```python
from build123d import *

# Parameters (mm, degrees)
SZKIC1_W                    = 30.3
SZKIC1_H                    = 11.1
SZKIC1_W_2                  = 28.304453741
SZKIC1_H_2                  = 9.1
DODANIE_WYCI_GNI_CIE1_DEPTH = 2
SZKIC2_W                    = 32.5
SZKIC2_H                    = 13.3
DODANIE_WYCI_GNI_CIE2_DEPTH = 1
ZAOKR_GLENIE1_R             = 0.5
SZKIC3_W                    = 1.095546259
SZKIC3_H                    = 0.5
SZKIC3_W_2                  = 1.2
SZKIC3_W_3                  = 0.5
SZKIC3_H_2                  = 1.2
SZKIC3_H_3                  = 1.1
WYTNIJ_WYCI_GNI_CIE1_DEPTH  = 1.4
ZAOKR_GLENIE2_R             = 0.5
SZKIC4_W                    = 2
SZKIC4_H                    = 1.15
SZKIC4_W_2                  = 1.145546259
SZKIC4_H_2                  = 2
SZKIC4_W_3                  = 1.15
DODANIE_WYCI_GNI_CIE3_DEPTH = 0.9
SZKIC5_W                    = 0.9
SZKIC5_H                    = 2
DODANIE_WYCI_GNI_CIE4_DEPTH = 0.5
SZKIC6_W                    = 2
SZKIC6_H                    = 0.9
DODANIE_WYCI_GNI_CIE5_DEPTH = 0.5
SZKIC7_W                    = 0.9
SZKIC7_H                    = 2
DODANIE_WYCI_GNI_CIE6_DEPTH = 0.5
ZAOKR_GLENIE5_R             = 1
SZKIC8_W                    = 28.304453741
SZKIC8_H                    = 9.1
DODANIE_WYCI_GNI_CIE7_DEPTH = 0.6
SZKIC9_W                    = 15.3
SZKIC9_H                    = 5.1
WYTNIJ_WYCI_GNI_CIE2_DEPTH  = 1.6
SZKIC10_W                   = 15.3
SZKIC10_H                   = 5.1
DODANIE_WYCI_GNI_CIE8_DEPTH = 2.5
ZAOKR_GLENIE6_R             = 0.4
SZKIC11_W                   = 2
SZKIC11_H                   = 5.1
WYTNIJ_WYCI_GNI_CIE3_DEPTH  = 0.3


with BuildPart() as part:
    # Szkic1 → Dodanie-wyciągnięcie1 (new body)
    with BuildSketch(Plane.XY):
        with Locations((-1.679789747, 1.465189223)):
            Rectangle(SZKIC1_W, SZKIC1_H)
        with Locations((-1.682016617, 1.465189223)):
            Rectangle(SZKIC1_W_2, SZKIC1_H_2, mode=Mode.SUBTRACT)
    extrude(amount=DODANIE_WYCI_GNI_CIE1_DEPTH)

    # Szkic2 → Dodanie-wyciągnięcie2 (add)
    with BuildSketch(Plane.XY.offset(2)):
        with Locations((-1.679789747, 1.465189223)):
            Rectangle(SZKIC2_W, SZKIC2_H)
    extrude(amount=DODANIE_WYCI_GNI_CIE2_DEPTH)

    # Zaokrąglenie1
    zaokr_glenie1_edges = [part.edges().sort_by_distance(p)[0] for p in [
        (-17.929789747, 1.465189223, 3),
        (-1.679789747, -5.184810777, 3),
        (14.570210253, 1.465189223, 3),
        (-1.679789747, 8.115189223, 3),
    ]]
    fillet(zaokr_glenie1_edges, radius=ZAOKR_GLENIE1_R)

    # Szkic3 → Wytnij-wyciągnięcie1 (cut)
    with BuildSketch(Plane(origin=(0, 0, 0), x_dir=(-1, 0, 0), z_dir=(0, 0, -1))):
        with Locations((16.382016617, 2.715189223)):
            Rectangle(SZKIC3_W, SZKIC3_H)
        with Locations((-13.070210253, 0.215189223)):
            Rectangle(SZKIC3_W_2, SZKIC3_H)
        with Locations((2.932016617, 6.615189223)):
            Rectangle(SZKIC3_W_3, SZKIC3_H_2)
        with Locations((0.432016617, 6.615189223)):
            Rectangle(SZKIC3_W_3, SZKIC3_H_2)
        with Locations((-13.070210253, 2.715189223)):
            Rectangle(SZKIC3_W_2, SZKIC3_H)
        with Locations((2.932016617, -3.634810777)):
            Rectangle(SZKIC3_W_3, SZKIC3_H_3)
        with Locations((0.432016617, -3.634810777)):
            Rectangle(SZKIC3_W_3, SZKIC3_H_3)
        with Locations((16.382016617, 0.215189223)):
            Rectangle(SZKIC3_W, SZKIC3_H)
    extrude(amount=-WYTNIJ_WYCI_GNI_CIE1_DEPTH, mode=Mode.SUBTRACT)

    # Zaokrąglenie2
    zaokr_glenie2_edges = [part.edges().sort_by_distance(p)[0] for p in [
        (6.644096818, 7.015189223, 0),
        (13.470210253, -2.059810777, 0),
        (-10.005903182, -4.084810777, 0),
        (-16.829789747, 4.990189223, 0),
        (-10.005903182, 7.015189223, 0),
        (13.470210253, 4.990189223, 0),
        (6.644096818, -4.084810777, 0),
        (-16.829789747, -2.059810777, 0),
    ]]
    fillet(zaokr_glenie2_edges, radius=ZAOKR_GLENIE2_R)

    # Szkic4 → Dodanie-wyciągnięcie3 (add)
    with BuildSketch(Plane(origin=(0, 0, 0), x_dir=(-1, 0, 0), z_dir=(0, 0, -1))):
        Polygon((0.682016617, 6.015189223), (2.682016617, 6.015189223), (2.682016617, 7.165189223), (2.682016617, 7.665189223), (0.682016617, 7.665189223), (0.682016617, 7.165189223), align=None)
        with Locations((1.682016617, -3.659810777)):
            Rectangle(SZKIC4_W, SZKIC4_H)
        with Locations((16.407016618, 1.465189223)):
            Rectangle(SZKIC4_W_2, SZKIC4_H_2)
        with Locations((-13.045210253, 1.465189223)):
            Rectangle(SZKIC4_W_3, SZKIC4_H_2)
    extrude(amount=-DODANIE_WYCI_GNI_CIE3_DEPTH)

    # Szkic5 → Dodanie-wyciągnięcie4 (add)
    with BuildSketch(Plane(origin=(13.620210253, 0, 0), x_dir=(0, 0, -1), z_dir=(1, 0, 0))):
        with Locations((-0.45, 1.465189223)):
            Rectangle(SZKIC5_W, SZKIC5_H)
    extrude(amount=DODANIE_WYCI_GNI_CIE4_DEPTH)

    # Szkic6 → Dodanie-wyciągnięcie5 (add)
    with BuildSketch(Plane.XZ.offset(4.234810777)):
        with Locations((-1.682016617, 0.45)):
            Rectangle(SZKIC6_W, SZKIC6_H)
    extrude(amount=DODANIE_WYCI_GNI_CIE5_DEPTH)

    # Szkic7 → Dodanie-wyciągnięcie6 (add)
    with BuildSketch(Plane.ZY.offset(16.979789747)):
        with Locations((0.45, 1.465189223)):
            Rectangle(SZKIC7_W, SZKIC7_H)
    extrude(amount=DODANIE_WYCI_GNI_CIE6_DEPTH)

    # Zaokrąglenie5
    # the kernel refuses this fillet: 1 mm, written as the material it takes off along each edge
    with BuildSketch(Plane(origin=(-5.16948521, 7.665189223, 0), x_dir=(0, -1, 0), z_dir=(1, 0, 0))) as zaokr_glenie5_piece_1:
        with BuildLine():
            CenterArc((0.994987437, -1), ZAOKR_GLENIE5_R, 90, 84.260829523)
            Line((0, -0.9), (-0.019899749, -0.898))
            ThreePointArc((-0.019899749, -0.898), (-0.02, -0.45), (-0.02, 0))
            Line((-0.02, 0), (0, 0.02))
            Line((0, 0.02), (0.994987437, 0.02))
            Line((0.994987437, 0.02), (0.994987437, 0))
        make_face()
    extrude(amount=6.974937186, mode=Mode.SUBTRACT)
    with BuildSketch(Plane(origin=(14.120210253, 4.952657816, 0), x_dir=(0, 0, 1), z_dir=(0, -1, 0)), Plane(origin=(1.805451975, -4.734810777, 0), x_dir=(0, 0, 1), z_dir=(-1, 0, 0)), Plane(origin=(-17.479789747, -2.02227937, 0), x_dir=(0, 0, 1), z_dir=(0, 1, 0))) as zaokr_glenie5_piece_2:
        with BuildLine():
            CenterArc((1, 0.994987437), ZAOKR_GLENIE5_R, 180, 84.260829523)
            Line((0, 0.994987437), (-0.02, 0.994987437))
            Line((-0.02, 0.994987437), (-0.02, 0))
            Line((-0.02, 0), (0, -0.02))
            ThreePointArc((0, -0.02), (0.45, -0.02), (0.898, -0.019899749))
            Line((0.898, -0.019899749), (0.9, 0))
        make_face()
    extrude(amount=6.974937186, mode=Mode.SUBTRACT)

    # Szkic8 → Dodanie-wyciągnięcie7 (add)
    with BuildSketch(Plane(origin=(0, 0, 2), x_dir=(-1, 0, 0), z_dir=(0, 0, -1))):
        with Locations((1.682016617, 1.465189223)):
            Rectangle(SZKIC8_W, SZKIC8_H)
    extrude(amount=DODANIE_WYCI_GNI_CIE7_DEPTH)

    # Szkic9 → Wytnij-wyciągnięcie2 (cut)
    with BuildSketch(Plane.XY.offset(3)):
        with Locations((-1.679789747, 1.465189223)):
            Rectangle(SZKIC9_W, SZKIC9_H)
    extrude(amount=-WYTNIJ_WYCI_GNI_CIE2_DEPTH, mode=Mode.SUBTRACT)

    # Szkic10 → Dodanie-wyciągnięcie8 (add)
    with BuildSketch(Plane(origin=(0, 0, 1.4), x_dir=(-1, 0, 0), z_dir=(0, 0, -1))):
        Polygon((-7.470210253, 5.515189223), (10.829789747, 5.515189223), (10.829789747, -2.584810777), (9.329789747, -2.584810777), (-5.970210253, -2.584810777), (-7.470210253, -2.584810777), align=None)
        with Locations((1.679789747, 1.465189223)):
            Rectangle(SZKIC10_W, SZKIC10_H, mode=Mode.SUBTRACT)
    extrude(amount=DODANIE_WYCI_GNI_CIE8_DEPTH)

    # Zaokrąglenie6
    zaokr_glenie6_edges = [part.edges().sort_by_distance(p)[0] for p in [
        (5.970210253, 1.465189223, -1.1),
        (-1.679789747, -1.084810777, -1.1),
        (-9.329789747, 1.465189223, -1.1),
        (-1.679789747, 4.015189223, -1.1),
    ]]
    fillet(zaokr_glenie6_edges, radius=ZAOKR_GLENIE6_R)

    # Szkic11 → Wytnij-wyciągnięcie3 (cut)
    with BuildSketch(Plane.XY.offset(3)):
        with Locations((-14.12705039, 1.465189223)):
            Rectangle(SZKIC11_W, SZKIC11_H)
    extrude(amount=-WYTNIJ_WYCI_GNI_CIE3_DEPTH, mode=Mode.SUBTRACT)


solid = part.part
```
For this review, take the finished solid that the model builds, in its own axes (mm). A direction names the side the tool comes from. Coordinates: 2 decimals unless noted, no trailing zeros. Order: outer loops, then holes, each group sorted by start corner. A loop starts at its lowest first (then second) coordinate and runs counter-clockwise, first axis right, second up. Notation, with made-up numbers: (42.25, 13.5) -> (69.25, 13.5) arc R17 ccw to (69.25, 29.5) -> close; hole circle Ø3 at (13, -6.75). An arc over 180 degrees is marked (long way). Answer as CSV lines item,"result".
Q1. For faces 1 (the face through (-0.182, -3.6, 0.7)), 2 (the face through (-16, 0.465, 1)), 3 (the face through (-3.182, 6.5, 0.7)), 4 (the face through (-14, 2, 2.7)), list the 3-axis set-ups (+Z, -Z, +X, -X, +Y, -Y) from which the entire face can be reached by the end or side of a thin tool; tool diameter is ignored.
Model answer:
face 1,"-Z, -Y"
face 2,"-Z, -X"
face 3,"-Z, +Y"
face 4,"+Z"
Q2. Clearance check with flat-ended pins moving along their axes: pin 1 Ø0.7 at (y, z) = (-2.5, 1) entering from -X; pin 2 Ø1 at (y, z) = (1, 0) entering from +X; pin 3 Ø1.6 at (x, z) = (-6, 1) entering from +Y. State where each tip first meets the part, or that it passes through.
Model answer:
pin 1,"stops at x = -16.83"
pin 2,"stops at x = 13.99"
pin 3,"stops at y = 7.02"
Q3. Draft analysis for pull direction X (two halves, no side actions). For faces 5 (the face through (6, 6.015, 1)), 6 (the face through (-16.83, 1.4, 1.2)), 7 (the face through (13, 2.465, 1)), state which applies: released by +X, released by -X, zero draft, split by the parting line, or undercut.
Model answer:
face 5,"undercut"
face 6,"released by -X"
face 7,"zero draft"
Q4. Wall thickness on line 1 along X through (y, z) = (3, 0.9); line 2 along X through (y, z) = (2.5, 0.65); line 3 along Y through (x, z) = (-2, -0.15): over which ranges is each line inside the solid? List them lowest first. Write a range as [from, to].
Model answer:
line 1,"x = [-16.83, -15.83], [-10.83, -9.33], [5.97, 7.47], [12.47, 13.47]"
line 2,"x = [-10.83, -9.33], [5.97, 7.47]"
line 3,"y = [-2.58, -1.08], [4.02, 5.52]"
Q5. We need section B-B (x = 1). State the section outline as (y, z) points.
Model answer:
outline,"(-5.18, 2) -> (-4.08, 2) -> (-4.08, 0.5) arc R0.5 ccw to (-3.58, 0) -> (-3.08, 0) -> (-3.08, 1.4) -> (-2.58, 1.4) -> (-2.58, -1.1) -> (-1.48, -1.1) arc R0.4 ccw to (-1.08, -0.7) -> (-1.08, 3) -> (-4.68, 3) arc R0.5 ccw to (-5.18, 2.5) -> close; (4.02, -0.7) arc R0.4 ccw to (4.42, -1.1) -> (5.52, -1.1) -> (5.52, 1.4) -> (6.02, 1.4) -> (6.02, 0) -> (6.52, 0) arc R0.5 ccw to (7.02, 0.5) -> (7.02, 2) -> (8.12, 2) -> (8.12, 2.5) arc R0.5 ccw to (7.62, 3) -> (4.02, 3) -> close"
Q6. We need section D-D (y = 5). State the section outline as (x, z) points, plus the area to 3 significant figures.
Model answer:
outline,"(-17.93, 2) -> (-16.83, 2) -> (-16.83, 0.5) arc R0.5 ccw to (-16.33, 0) -> (-15.83, 0) -> (-15.83, 1.4) -> (-10.83, 1.4) -> (-10.83, -1.1) -> (7.47, -1.1) -> (7.47, 1.4) -> (12.47, 1.4) -> (12.47, 0) -> (12.97, 0) arc R0.5 ccw to (13.47, 0.5) -> (13.47, 2) -> (14.57, 2) -> (14.57, 2.5) arc R0.5 ccw to (14.07, 3) -> (-17.43, 3) arc R0.5 ccw to (-17.93, 2.5) -> close"
area,"99.0 mm2"
Q7. We need section C-C (z = -0.4). State the section outline as (x, y) points, plus the area to 3 significant figures.
Model answer:
outline,"(-10.83, -2.58) -> (7.47, -2.58) -> (7.47, 5.52) -> (-10.83, 5.52) -> close; hole (-9.33, -1.08) -> (5.97, -1.08) -> (5.97, 4.02) -> (-9.33, 4.02) -> close"
area,"70.2 mm2"
